```python
from build123d import *

# Parameters (mm, degrees)
F1_R      = 23.5
F2_DEPTH  = 23
F3_R      = 22.99999
F0_W      = 32
F0_H      = 31.9999990161
F4_DEPTH  = 3
F5_R      = 2.25
F6_DEPTH  = 8
F7_W      = 12.7981919795
F7_H      = 23.941071704
F8_DEPTH  = 23.001
F9_W      = 11.722983385
F9_H      = 16.8361999094
F10_DEPTH = 13


# Not quite as in the source:
# - a fillet or chamfer is up to 0.001 mm smaller than in the source, because OpenCascade refuses the exact size


with BuildPart() as f2:
    # F1 (on Right) → F2 (new body)
    with BuildSketch(Plane.YZ):
        Circle(F1_R)
    extrude(amount=F2_DEPTH)

    # F3 (radius 23 in the source; OpenCascade refuses exactly that, so slightly less here)
    f3_edges = [f2.edges().sort_by_distance(p)[0] for p in [
        (23, -23.5, 0),
    ]]
    fillet(f3_edges, radius=F3_R)

    # F0 (on Right) → F4 (cut)
    with BuildSketch(Plane.YZ):
        with Locations((-0.437150538, 0.2656796428)):
            Rectangle(F0_W, F0_H)
    extrude(amount=F4_DEPTH, mode=Mode.SUBTRACT)

    # F5 (on Right) → F6 (cut)
    with BuildSketch(Plane.YZ):
        with Locations((18.515, 0)):
            Circle(F5_R)
        with Locations((-19.4516796619, 0)):
            Circle(F5_R)
    extrude(amount=F6_DEPTH, mode=Mode.SUBTRACT)

    # F7 (on face) → F8 (cut, through all)
    with BuildSketch(Plane.YZ):
        with Locations((8.9887827635, 4.0837647393)):
            Rectangle(F7_W, F7_H)
    extrude(amount=F8_DEPTH, mode=Mode.SUBTRACT)

    # F9 (on Right) → F10 (cut)
    with BuildSketch(Plane.YZ):
        with Locations((-6.7771898757, 4.8962011933)):
            Rectangle(F9_W, F9_H)
    extrude(amount=F10_DEPTH, mode=Mode.SUBTRACT)


solid = f2.part
```
Read the model definition and answer for the solid it produces. Units are mm, in the model's axes. A direction names the side the tool comes from. Coordinates: 2 decimals unless noted, no trailing zeros. Return JSON: item names as keys, results as strings.
1. Each of these flat-tipped pins is pushed along its axis until it touches: P1, Ø5, axis at x = 16.5, y = -10, coming from the -Z side; P2, Ø3.5, axis at y = -19.45, z = 0, coming from the -X side; P3, Ø12, axis at x = 20, z = -2.5, coming from the -Y side; P4, Ø6, axis at y = 17.5, z = -0.5, coming from the -X side. Where does it stop, or does it pass through?
Found:
{"P1": "z = -16.28", "P2": "x = 8", "P3": "y = -18.63", "P4": "x = 0"}
2. Find the intervals of material crossed by line 1 along Y through (x, z) = (8.25, 6); line 2 along Y through (x, z) = (2.5, -2.5); line 3 along Y through (x, z) = (5, 1), in increasing order. Write a range as from..to.
Found:
{"line 1": "-21.13..-12.64, -0.92..2.59, 15.39..21.13", "line 2": "-23.23..-16.44, 15.56..23.23", "line 3": "-22.93..-21.47, -17.44..-12.64, -0.92..2.59, 15.39..16.5, 20.53..22.93"}
3. A tool of negligible diameter and unlimited length cuts with its end or side. For faces 3 (the face through (12, 9, -7.887)), 4 (the face through (8, -7, -3.522)), from which of +Z, -Z, +X, -X, +Y, -Y can it reach the whole face along a straight path? Write none if from no direction.
Found:
{"face 3": "+X, -X", "face 4": "-X"}
4. Determine the mould class of faces 1 (the face through (0, 2, -17)), 2 (the face through (1, -16.437, 0)) for opening direction Z: pulls with the +Z half, pulls with the -Z half, needs draft (parallel to the pull), parting line crosses it, or undercut.
Found:
{"face 1": "needs draft", "face 2": "undercut"}
